```python
from build123d import *

# Parameters (mm, degrees)
BOSS_EXTRUDE1_DEPTH = 3.683
SKETCH2_W           = 46.355
SKETCH2_H           = 26.797
BOSS_EXTRUDE2_DEPTH = 10.287


with BuildPart() as part:
    # Sketch1 → Boss-Extrude1 (new body)
    with BuildSketch(Plane(origin=(0, 0, 0), x_dir=(1, 0, 0), z_dir=(0, 1, 0))):
        with BuildLine():
            Line((0, 0), (46.355, 0))
            Line((46.355, 0), (46.355, 5.945116694))
            ThreePointArc((46.355, 5.945116694), (46.428176367, 6.169628633), (46.619596382, 6.307899271))
            Line((46.619596382, 6.307899271), (55.1815, 9.0551))
            Line((55.1815, 9.0551), (55.1815, 11.5951))
            Line((55.1815, 11.5951), (47.9298, 11.5951))
            ThreePointArc((47.9298, 11.5951), (46.816248241, 12.056348241), (46.355, 13.1699))
            Line((46.355, 13.1699), (46.355, 13.6271))
            ThreePointArc((46.355, 13.6271), (46.816248241, 14.740651759), (47.9298, 15.2019))
            Line((47.9298, 15.2019), (55.1815, 15.2019))
            Line((55.1815, 15.2019), (55.1815, 17.7419))
            Line((55.1815, 17.7419), (46.619596382, 20.489100729))
            ThreePointArc((46.619596382, 20.489100729), (46.428176367, 20.627371367), (46.355, 20.851883306))
            Line((46.355, 20.851883306), (46.355, 26.797))
            Line((46.355, 26.797), (0, 26.797))
            Line((0, 26.797), (0, 20.851883306))
            ThreePointArc((0, 20.851883306), (-0.073176367, 20.627371367), (-0.264596382, 20.489100729))
            Line((-0.264596382, 20.489100729), (-8.8265, 17.7419))
            Line((-8.8265, 17.7419), (-8.8265, 15.2019))
            Line((-8.8265, 15.2019), (-1.5748, 15.2019))
            ThreePointArc((-1.5748, 15.2019), (-0.461248241, 14.740651759), (0, 13.6271))
            Line((0, 13.6271), (0, 13.1699))
            ThreePointArc((0, 13.1699), (-0.461248241, 12.056348241), (-1.5748, 11.5951))
            Line((-1.5748, 11.5951), (-8.8265, 11.5951))
            Line((-8.8265, 11.5951), (-8.8265, 9.0551))
            Line((-8.8265, 9.0551), (-0.264596382, 6.307899271))
            ThreePointArc((-0.264596382, 6.307899271), (-0.073176367, 6.169628633), (0, 5.945116694))
            Line((0, 5.945116694), (0, 0))
        make_face()
    extrude(amount=BOSS_EXTRUDE1_DEPTH)

    # Sketch2 → Boss-Extrude2 (add)
    with BuildSketch(Plane(origin=(0, 3.683, 0), x_dir=(1, 0, 0), z_dir=(0, 1, 0))):
        with Locations((23.1775, 13.3985)):
            Rectangle(SKETCH2_W, SKETCH2_H)
    extrude(amount=BOSS_EXTRUDE2_DEPTH)


solid = part.part
```
Input: part model. Units: mm. Frame: model coordinates. A direction names the side the tool comes from. Give positions to 0.01 mm unless a question says otherwise; leave off trailing zeros. Loops run counter-clockwise (first coordinate to the right, second up) from the corner with the lowest first, then second, coordinate; pieces in that order, holes last. Notation, with made-up numbers: M -33,47 L -4,47 A23 ccw -4,75 Z; hole C -1.5,59.25 d9. An arc over 180 degrees is marked long. Answer as CSV lines item,"result". Start each with the question number.
1. Section A-A on z = -10.5. Return loops of the section in (x, y) (1 decimal), plus the area to 3 significant figures.
2. Reachability of faces 5 (the face through (46.83, 1.82, -12.04)), 6 (the face through (-4, 3.683, -10)), 7 (the face through (-0.47, 1.82, -14.75)) from +Z, -Z, +X, -X, +Y, -Y: full face, straight path, thin tool, end or side. Return the list, or none.
3. Pull-direction query (Z, two-part tool) for faces 1 (the face through (46.804, 1.816, -14.728)), 2 (the face through (50.96, 1.816, -19.096)), 3 (the face through (-8.826, 2, -10)), 4 (the face through (-5, 2, -15.202)); classes: released by +Z, released by -Z, zero draft, split by the parting line, or undercut.
4. Section C-C on z = -4. Return loops of the section in (x, y) (3 decimals).
5. Section B-B on y = 2.5. Return loops of the section in (x, z) (1 decimal).
6. Line query: L1, parallel to X at y = 3, z = -24.5 (3 decimals); L2, parallel to Z at x = -5, y = 1.25; L3, parallel to Y at x = 47, z = -6.5. Output: solid intervals per line, ascending.
7. Pin query (flat end, axial travel): P1, Ø1.8, axis at x = 51.5, y = 1, coming from the -Z side; P2, Ø6, axis at x = 52, z = -18, coming from the +Y side; P3, Ø1.8, axis at x = 52, y = 1.5, coming from the +Z side. Return the tip coordinate at first contact, or that it passes through.
8. Section D-D on y = 8.5. Return loops of the section in (x, z) (3 decimals), plus the area to 3 significant figures.
Computed values:
1,outline,"M -8.8,0 L 55.2,0 L 55.2,3.7 L 46.4,3.7 L 46.4,14 L 0,14 L 0,3.7 L -8.8,3.7 Z"
1,area,"713 mm²"
2,face 5,"+X, +Y, -Y"
2,face 6,"+Z, -Z, -X, +Y"
2,face 7,"-X, +Y, -Y"
3,face 1,"undercut"
3,face 2,"released by -Z"
3,face 3,"zero draft"
3,face 4,"undercut"
4,outline,"M 0,0 L 46.355,0 L 46.355,13.97 L 0,13.97 Z"
5,outline,"M -8.8,-17.7 L -0.3,-20.5 A0.4 cw 0,-20.9 L 0,-26.8 L 46.4,-26.8 L 46.4,-20.9 A0.4 cw 46.6,-20.5 L 55.2,-17.7 L 55.2,-15.2 L 47.9,-15.2 A1.6 cw 46.4,-13.6 L 46.4,-13.2 A1.6 cw 47.9,-11.6 L 55.2,-11.6 L 55.2,-9.1 L 46.6,-6.3 A0.4 cw 46.4,-5.9 L 46.4,0 L 0,0 L 0,-5.9 A0.4 cw -0.3,-6.3 L -8.8,-9.1 L -8.8,-11.6 L -1.6,-11.6 A1.6 cw 0,-13.2 L 0,-13.6 A1.6 cw -1.6,-15.2 L -8.8,-15.2 Z"
6,L1,"x = 0 to 46.355"
6,L2,"z = -18.97 to -15.2, -11.6 to -7.83"
6,L3,"y = 0 to 3.68"
7,P1,"stops at z = -19.21"
7,P2,"stops at y = 3.68"
7,P3,"stops at z = -7.75"
8,outline,"M 0,-26.797 L 46.355,-26.797 L 46.355,0 L 0,0 Z"
8,area,"1,240 mm²"
